For this review, take the finished solid that the model builds, in its own axes (mm). A direction names the side the tool comes from. Give positions to 0.01 mm unless a question says otherwise; leave off trailing zeros. Write each loop counter-clockwise with the first axis right and the second up, starting at its lowest first coordinate (ties: lowest second). Pieces come first, ordered by that corner, then holes. Notation, with made-up numbers: M 75.25,-11.5 L 108.25,-11.5 A15 ccw 108.25,-4.5 Z; hole C 32,47 d2. An arc over 180 degrees is marked long. Use one line per item in the form item = value. Start each with the question number.
Q1. Consider section D-D on x = 48.5. Write out the cut boundary in (y, z).
Q2. Consider section A-A on y = -5. Write out the cut boundary in (x, z), and give its area (3 significant figures).
Q3. Mouldability with a two-part tool opening along Z and no side actions: class faces 1 (the flat face through (3, -57, 12)), 2 (the flat face through (41, -38, 4)), 3 (the cylindrical face through (81, -5, 14)) as released by +Z, released by -Z, zero draft, split by the parting line, or undercut.
Q4. Consider section C-C on y = -58.5. Write out the cut boundary in (x, z), and give its area (3 significant figures).
Q5. Tool access review of faces 4 (the flat face through (67.55, -51.29, 11.67)), 5 (the flat face through (3, -3, 12)), 6 (the flat face through (40, 0, 8)): name each direction out of +Z, -Z, +X, -X, +Y, -Y from which nothing blocks a thin tool from reaching the whole face with its end or side.
Q6. Consider section B-B on x = 5. Write out the cut boundary in (y, z).
Q7. Clearance check with flat-ended pins moving along their axes: pin 1 Ø8 at (x, z) = (48.5, 5) entering from -Y; pin 2 Ø4 at (x, y) = (4, -59.5) entering from +Z; pin 3 Ø3 at (x, z) = (42, 5) entering from +Y. State where each tip first meets the part, or that it passes through.
Q8. For probe 1 along Y at (x, z) = (77, 6); probe 2 along X at (y, z) = (-58.5, 13.1); probe 3 along X at (y, z) = (-50, 5.25), list the stretches that pass through material, from the lowest coordinate up. Write a range as [from, to].
```python
from build123d import *

# Parameters (mm, degrees)
SKETCH_1_W                  = 82
SKETCH_1_H                  = 63.5
EXTRUDE_1_DEPTH             = 16
CUT_EXTRUDE_1_DEPTH         = 83
SKETCH_15_W                 = 25
SKETCH_15_H                 = 14.711451884
CUT_EXTRUDE_4_DEPTH         = 7
SKETCH_16_W                 = 25
SKETCH_16_H                 = 10.67
CUT_EXTRUDE_5_DEPTH         = 9
SKETCH_17_R                 = 2.5
CUT_EXTRUDE_6_DEPTH         = 4
M4X0_72_D                   = 3.3
M4X0_72_DEPTH               = 10
M4X0_72_TIP                 = 0.991420021
CUT_EXTRUDE_7_DEPTH         = 4
SKETCH_26_R                 = 3.25
CUT_EXTRUDE_8_DEPTH         = 38
HOLE_WIZARD_M41_D           = 4.5
HOLE_WIZARD_M41_CBORE_D     = 8
HOLE_WIZARD_M41_CBORE_DEPTH = 4
CHAMFER_2_SIZE              = 1
CHAMFER_2_SIZE2             = 2
CHAMFER_2_PART_2_SIZE       = 1
CHAMFER_2_PART_2_SIZE2      = 2
CHAMFER_2_PART_3_SIZE       = 1
CHAMFER_2_PART_3_SIZE2      = 2


with BuildPart() as part:
    # Эскиз1 → Бобышка-Вытянуть1 (new body)
    with BuildSketch(Plane.XY):
        with Locations((41, -31.75)):
            Rectangle(SKETCH_1_W, SKETCH_1_H)
    extrude(amount=EXTRUDE_1_DEPTH)

    # Эскиз2 → Вырез-Вытянуть1 (cut, through all)
    with BuildSketch(Plane.ZY):
        Polygon((9, -10.67), (16, -14.711451884), (16, -48.788548116), (9, -52.83), align=None)
    extrude(amount=-CUT_EXTRUDE_1_DEPTH, mode=Mode.SUBTRACT)

    # Эскиз15 → Вырез-Вытянуть4 (cut)
    with BuildSketch(Plane.XY.offset(16)):
        with Locations((41, -56.144274058)):
            Rectangle(SKETCH_15_W, SKETCH_15_H)
    extrude(amount=-CUT_EXTRUDE_4_DEPTH, mode=Mode.SUBTRACT)

    # Эскиз16 → Вырез-Вытянуть5 (cut)
    with BuildSketch(Plane.XY.offset(9)):
        with Locations((41, -58.165)):
            Rectangle(SKETCH_16_W, SKETCH_16_H)
    extrude(amount=-CUT_EXTRUDE_5_DEPTH, mode=Mode.SUBTRACT)

    # Эскиз17 → Вырез-Вытянуть6 (cut)
    with BuildSketch(Plane.XZ.offset(52.83)):
        with Locations((33.5, 5)):
            Circle(SKETCH_17_R)
        with Locations((48.5, 5)):
            Circle(SKETCH_17_R)
    extrude(amount=-CUT_EXTRUDE_6_DEPTH, mode=Mode.SUBTRACT)

    # Отверстие обработанное метчиком M4x0.72
    with Locations(Plane(origin=(0, -52.83, 0), x_dir=(-1, 0, 0), z_dir=(0, -1, 0))):
        with Locations((-41, -5)):
            Hole(M4X0_72_D / 2, depth=M4X0_72_DEPTH)
            with Locations((0, 0, -(M4X0_72_DEPTH + M4X0_72_TIP / 2))):  # 118° drill point
                Cone(0, M4X0_72_D / 2, M4X0_72_TIP, mode=Mode.SUBTRACT)

    # Эскиз25 → Вырез-Вытянуть7 (cut)
    with BuildSketch(Plane.XY.offset(9)):
        with BuildLine():
            Line((44.1, -18.711451884), (44.1, -25.711451884))
            ThreePointArc((44.1, -25.711451884), (41, -28.811451884), (37.9, -25.711451884))
            Line((37.9, -25.711451884), (37.9, -18.711451884))
            ThreePointArc((37.9, -18.711451884), (41, -15.611451884), (44.1, -18.711451884))
        make_face()
    extrude(amount=-CUT_EXTRUDE_7_DEPTH, mode=Mode.SUBTRACT)

    # Эскиз26 → Вырез-Вытянуть8 (cut)
    with BuildSketch(Plane(origin=(0, 0, 0), x_dir=(1, 0, 0), z_dir=(0, 1, 0))):
        with Locations((41, -4.5)):
            Circle(SKETCH_26_R)
    extrude(amount=-CUT_EXTRUDE_8_DEPTH, mode=Mode.SUBTRACT)

    # Цековка для винта с внутренним шестигранником M41 (through all)
    with Locations(Plane(origin=(30.759227947, 26.793365177, 16), x_dir=(-1, 0, 0), z_dir=(0, 0, 1))):
        with Locations((-46.240772053, 31.793365177), (-46.240772053, 85.293365177), (25.759227947, 85.293365177), (25.759227947, 31.793365177)):
            CounterBoreHole(HOLE_WIZARD_M41_D / 2, HOLE_WIZARD_M41_CBORE_D / 2, HOLE_WIZARD_M41_CBORE_DEPTH)

    # Фаска2
    chamfer_2_edges = [part.edges().sort_by_distance(p)[0] for p in [
        (41, -14.711451884, 16),
    ]]
    chamfer_2_side = [part.faces().sort_by_distance(p)[0] for p in [
        (41, -7.569889145, 16),
    ]]
    chamfer(chamfer_2_edges, length=CHAMFER_2_SIZE, length2=CHAMFER_2_SIZE2, reference=chamfer_2_side[0])

    # Фаска2 part 2
    chamfer_2_part_2_edges = [part.edges().sort_by_distance(p)[0] for p in [
        (67.75, -48.788548116, 16),
    ]]
    chamfer_2_part_2_side = [part.faces().sort_by_distance(p)[0] for p in [
        (66.489994625, -55.823384615, 16),
    ]]
    chamfer(chamfer_2_part_2_edges, length=CHAMFER_2_PART_2_SIZE, length2=CHAMFER_2_PART_2_SIZE2, reference=chamfer_2_part_2_side[0])

    # Фаска2 part 3
    chamfer_2_part_3_edges = [part.edges().sort_by_distance(p)[0] for p in [
        (14.25, -48.788548116, 16),
    ]]
    chamfer_2_part_3_side = [part.faces().sort_by_distance(p)[0] for p in [
        (15.510005375, -55.823384615, 16),
    ]]
    chamfer(chamfer_2_part_3_edges, length=CHAMFER_2_PART_3_SIZE, length2=CHAMFER_2_PART_3_SIZE2, reference=chamfer_2_part_3_side[0])


solid = part.part
```
Working result:
q1.outline = M -52.83,0 L 0,0 L 0,16 L -13.71,16 L -13.71,14.27 L -10.67,9 L -52.83,9 L -52.83,7.5 L -48.83,7.5 L -48.83,2.5 L -52.83,2.5 Z
q2.outline = M 0,0 L 2.75,0 L 2.75,12 L 1,12 L 1,16 L 0,16 Z; M 7.25,0 L 74.75,0 L 74.75,12 L 73,12 L 73,16 L 9,16 L 9,12 L 7.25,12 Z; M 79.25,0 L 82,0 L 82,16 L 81,16 L 81,12 L 79.25,12 Z; hole C 41,4.5 d6.5
q2.area = 1,110 mm²
q3.face_1 = released by +Z
q3.face_2 = undercut
q3.face_3 = zero draft
q4.outline = M 0,0 L 2.75,0 L 2.75,12 L 1,12 L 1,16 L 0,16 Z; M 7.25,0 L 28.5,0 L 28.5,16 L 9,16 L 9,12 L 7.25,12 Z; M 53.5,0 L 74.75,0 L 74.75,12 L 73,12 L 73,16 L 53.5,16 Z; M 79.25,0 L 82,0 L 82,16 L 81,16 L 81,12 L 79.25,12 Z
q4.area = 740 mm²
q5.face_4 = +X, -X
q5.face_5 = +Z
q5.face_6 = +Z, -Z, +X, -X, +Y
q6.outline = M -63.5,0 L -60.75,0 L -60.75,12 L -62.5,12 L -62.5,16 L -63.5,16 Z; M -56.25,0 L -7.25,0 L -7.25,12 L -9,12 L -9,16 L -13.71,16 L -13.71,14.27 L -10.67,9 L -52.83,9 L -49.79,14.27 L -49.79,16 L -54.5,16 L -54.5,12 L -56.25,12 Z; M -2.75,0 L 0,0 L 0,16 L -1,16 L -1,12 L -2.75,12 Z
q7.pin_1 = -52.83
q7.pin_2 = 12
q7.pin_3 = -38
q8.probe_1 = [-63.5, -60.75], [-56.25, -7.25], [-2.75, 0]
q8.probe_2 = [0, 1], [9, 28.5], [53.5, 73], [81, 82]
q8.probe_3 = [0, 31.01], [35.99, 39.37], [42.63, 46.01], [50.99, 82]
